```python
from build123d import *

# Parameters (mm, degrees)
F0_R           = 15.25
F1_DEPTH       = 9.5
F2_R           = 30
F3_DEPTH       = 3
F4_DEPTH       = 3
F5_DEPTH       = 3
F6_D           = 8
F6_DEPTH       = 5
F6_TIP         = 2.4034424761
F7_D           = 8
F7_DEPTH       = 5
F7_TIP         = 2.4034424761
F8_D           = 8
F8_DEPTH       = 5
F8_TIP         = 2.4034424761
F9_D           = 20
F9_DEPTH       = 50
F9_CBORE_D     = 27.5
F9_CBORE_DEPTH = 6.5
F9_TIP         = 6.0086061903


with BuildPart() as f1:
    # F0 (on Top) → F1 (new body)
    with BuildSketch(Plane.XY):
        Circle(F0_R)
    extrude(amount=F1_DEPTH)



with BuildPart() as f3:
    # F2 (on face) → F3 (new body)
    with BuildSketch(Plane.XY.offset(9.5)):
        Circle(F2_R)
        with BuildLine():
            ThreePointArc((0, 22.5), (15.9099025767, 15.9099025767), (22.5, 0))
            ThreePointArc((22.5, 0), (21.7333310915, -5.8234285148), (19.4855715851, -11.25))
            ThreePointArc((19.4855715851, -11.25), (0, -22.5), (-19.4855715851, -11.25))
            ThreePointArc((-19.4855715851, -11.25), (-19.4855715851, 11.25), (0, 22.5))
        make_face(mode=Mode.SUBTRACT)
    extrude(amount=-F3_DEPTH)


with BuildPart() as f1_1:
    add(f1.part)

    add(f3.part)  # F3#2 merges F3
    # F2 (on face) → F3, piece 2 (join)
    with BuildSketch(Plane.XY.offset(9.5)):
        with BuildLine():
            Line((-14.8906008631, -3.2912772501), (-19.4855715851, -11.25))
            Line((-19.4855715851, -11.25), (-10.295630141, -11.25))
            ThreePointArc((-10.295630141, -11.25), (-13.2068874077, -7.625), (-14.8906008631, -3.2912772501))
        make_face()
    extrude(amount=-F3_DEPTH)

    # F2 (on face) → F4 (join)
    with BuildSketch(Plane.XY.offset(9.5)):
        with BuildLine():
            Line((-4.5949707221, 14.5412772501), (0, 22.5))
            ThreePointArc((0, 22.5), (-19.4855715851, 11.25), (-19.4855715851, -11.25))
            Line((-19.4855715851, -11.25), (-14.8906008631, -3.2912772501))
            ThreePointArc((-14.8906008631, -3.2912772501), (-13.2068874077, 7.625), (-4.5949707221, 14.5412772501))
        make_face()
        with BuildLine():
            ThreePointArc((-19.4855715851, -11.25), (0, -22.5), (19.4855715851, -11.25))
            Line((19.4855715851, -11.25), (10.295630141, -11.25))
            ThreePointArc((10.295630141, -11.25), (0, -15.25), (-10.295630141, -11.25))
            Line((-10.295630141, -11.25), (-19.4855715851, -11.25))
        make_face()
        with BuildLine():
            ThreePointArc((19.4855715851, -11.25), (21.7333310915, -5.8234285148), (22.5, 0))
            ThreePointArc((22.5, 0), (15.9099025767, 15.9099025767), (0, 22.5))
            Line((0, 22.5), (4.5949707221, 14.5412772501))
            ThreePointArc((4.5949707221, 14.5412772501), (12.3011341654, 9.0135785482), (15.25, 0))
            ThreePointArc((15.25, 0), (15.1598839567, -1.655420919), (14.8906008631, -3.2912772501))
            Line((14.8906008631, -3.2912772501), (19.4855715851, -11.25))
        make_face()
    extrude(amount=-F4_DEPTH)

    # F2 (on face) → F5 (join)
    with BuildSketch(Plane.XY.offset(9.5)):
        with BuildLine():
            Line((4.5949707221, 14.5412772501), (0, 22.5))
            Line((0, 22.5), (-4.5949707221, 14.5412772501))
            ThreePointArc((-4.5949707221, 14.5412772501), (0, 15.25), (4.5949707221, 14.5412772501))
        make_face()
        with BuildLine():
            ThreePointArc((-19.4855715851, -11.25), (0, -22.5), (19.4855715851, -11.25))
            Line((19.4855715851, -11.25), (10.295630141, -11.25))
            ThreePointArc((10.295630141, -11.25), (0, -15.25), (-10.295630141, -11.25))
            Line((-10.295630141, -11.25), (-19.4855715851, -11.25))
        make_face()
        with BuildLine():
            Line((10.295630141, -11.25), (19.4855715851, -11.25))
            Line((19.4855715851, -11.25), (14.8906008631, -3.2912772501))
            ThreePointArc((14.8906008631, -3.2912772501), (13.2068874077, -7.625), (10.295630141, -11.25))
        make_face()
    extrude(amount=-F5_DEPTH)

    # F6
    with Locations(Plane.XY.offset(9.5)):
        with Locations((-19.4855715851, -11.25)):
            Hole(F6_D / 2, depth=F6_DEPTH)
            with Locations((0, 0, -(F6_DEPTH + F6_TIP / 2))):  # 118° drill point
                Cone(0, F6_D / 2, F6_TIP, mode=Mode.SUBTRACT)

    # F7
    with Locations(Plane.XY.offset(9.5)):
        with Locations((0, 22.5)):
            Hole(F7_D / 2, depth=F7_DEPTH)
            with Locations((0, 0, -(F7_DEPTH + F7_TIP / 2))):  # 118° drill point
                Cone(0, F7_D / 2, F7_TIP, mode=Mode.SUBTRACT)

    # F8
    with Locations(Plane.XY.offset(9.5)):
        with Locations((19.4855715851, -11.25)):
            Hole(F8_D / 2, depth=F8_DEPTH)
            with Locations((0, 0, -(F8_DEPTH + F8_TIP / 2))):  # 118° drill point
                Cone(0, F8_D / 2, F8_TIP, mode=Mode.SUBTRACT)

    # F9
    with Locations(Plane.XY.offset(9.5)):
        with Locations((0, 0)):
            CounterBoreHole(F9_D / 2, F9_CBORE_D / 2, F9_CBORE_DEPTH, depth=F9_DEPTH)
            with Locations((0, 0, -(F9_DEPTH + F9_TIP / 2))):  # 118° drill point
                Cone(0, F9_D / 2, F9_TIP, mode=Mode.SUBTRACT)


solid = f1_1.part
```
Model file for the job. Use its own axes, mm. A direction names the side the tool comes from. Round coordinates to 2 decimals unless told otherwise and drop trailing zeros. Order: outer loops, then holes, each group sorted by start corner. A loop starts at its lowest first (then second) coordinate and runs counter-clockwise, first axis right, second up. Notation, with made-up numbers: (69, 44.25) -> (83, 44.25) arc R20 cw to (83, 57.25) -> close; hole circle Ø5 at (68.5, 19.5). An arc over 180 degrees is marked (long way). Use one line per item in the form item = value.
Item 1: Tool access for faces 4 (the face through (-23.18, -12.78, 7.98)), 5 (the face through (-2.981, -13.423, 6.296)), 6 (the face through (-12.1, -9.28, 3.2)): list every direction of +Z, -Z, +X, -X, +Y, -Y with a clear straight run to the whole face (end or side of a thin tool).
Returned:
face_4 = +Z, -Z
face_5 = +Z
face_6 = -Z
Item 2: Drill centre lines: line 1 (Y direction, x = 0, z = 0.6); line 2 (Z direction, x = -17, y = 16.5); line 3 (Y direction, x = 5, z = 3.5). Where is each one in solid material? Low to high.
Returned:
line_1 = -15.25 to -10, 10 to 15.25
line_2 = 6.5 to 9.5
line_3 = -14.41 to -12.81, 12.81 to 14.41
Item 3: Cut at A-A, the plane y = 0. Write the cut outline in (x, z), and give its area (4 significant figures).
Returned:
outline = (-30, 6.5) -> (-15.25, 6.5) -> (-15.25, 0) -> (-10, 0) -> (-10, 3) -> (-13.75, 3) -> (-13.75, 9.5) -> (-30, 9.5) -> close; (10, 0) -> (15.25, 0) -> (15.25, 6.5) -> (30, 6.5) -> (30, 9.5) -> (13.75, 9.5) -> (13.75, 3) -> (10, 3) -> close
area = 139.5 mm^2
Item 4: Pull direction Y, two halves, no side cores. Call faces 1 (the face through (13, -6, 9.5)), 2 (the face through (0.95, -10.12, 3)), 3 (the face through (-29.97, 1.32, 8.02)): released by +Y, released by -Y, zero draft, split by the parting line, or undercut.
Returned:
face_1 = zero draft
face_2 = undercut
face_3 = split by the parting line
Item 5: Cut at D-D, the plane z = 8.25. Write the cut outline in (x, y).
Returned:
outline = circle Ø60 at (0, 0); hole circle Ø8 at (-19.49, -11.25); hole circle Ø27.5 at (0, 0); hole circle Ø8 at (0, 22.5); hole circle Ø8 at (19.49, -11.25)
Item 6: Cut at C-C, the plane x = -22. Write the cut outline in (y, z), and give its area (3 significant figures).
Returned:
outline = (-20.4, 6.5) -> (-14.36, 6.5) -> (-14.36, 9.5) -> (-20.4, 9.5) -> close; (-8.14, 6.5) -> (20.4, 6.5) -> (20.4, 9.5) -> (-8.14, 9.5) -> close
area = 104 mm^2
Item 7: Flat gauge pins, fed straight in: pin 1 Ø22 at (x, y) = (0.5, -2) entering from +Z; pin 2 Ø7 at (x, y) = (0, 22.5) entering from -Z; pin 3 Ø5 at (y, z) = (2, 1) entering from +X; pin 4 Ø3 at (y, z) = (5.5, 2) entering from -X. Where does each tip first touch, or does it go through?
Returned:
pin_1 = 3
pin_2 = through
pin_3 = 15.25
pin_4 = -14.72
Item 8: Cut at B-B, the plane x = 0. Write the cut outline in (y, z), and give its area (4 significant figures).
Returned:
outline = (-30, 6.5) -> (-15.25, 6.5) -> (-15.25, 0) -> (-10, 0) -> (-10, 3) -> (-13.75, 3) -> (-13.75, 9.5) -> (-30, 9.5) -> close; (10, 0) -> (15.25, 0) -> (15.25, 6.5) -> (18.5, 6.5) -> (18.5, 9.5) -> (13.75, 9.5) -> (13.75, 3) -> (10, 3) -> close; (26.5, 6.5) -> (30, 6.5) -> (30, 9.5) -> (26.5, 9.5) -> close
area = 115.5 mm^2
